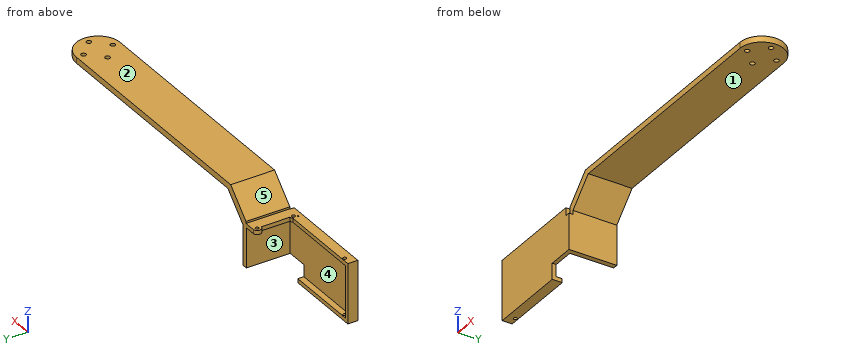
Autodesk Inventor part; units mm, degrees
ref_plane "YZ Plane" through (0, 0, 0) normal (1, 0, 0) x (0, 1, 0)
ref_plane "XZ Plane" through (0, 0, 0) normal (0, 1, 0) x (-1, 0, 0)
ref_plane "XY Plane" through (0, 0, 0) normal (0, 0, 1) x (1, 0, 0)
ref_plane "Plano de trabajo1" through (0, 0, 0) normal (0, 0, 1) x (1, 0, 0)
sketch "Boceto1" plane through (0, 0, 0) normal (0, 0, 1) x (1, 0, 0)
  circle A0 centre (10.9923, -7.35) radius 1.2028
  circle A1 centre (3.6423, 0) radius 1.2028
  circle A2 centre (18.3423, 0) radius 1.2028
  circle A3 centre (10.9923, 7.35) radius 1.2028
  circle A4 centre (10.9923, 0) radius 10.9823
  line L0 (10.9923, -10.9823) -> (-139.0077, -10.9823)
  line L1 (10.9923, 10.9823) -> (-139.0077, 10.9823)
  line L2 (-139.0077, 10.9823) -> (-139.0077, -10.9823)
  point P0 (0, 0)
  dimension "d0" = 150
  dimension "d1" = 150
extrude "Extrusión1" add sketch "Boceto1" along normal blind 3
sketch "Boceto2" plane through (0, 0, 3) normal (0, 0, 1) x (1, 0, 0)
  arc A0 (-129.1978, -5.6745) -> (-132.1454, -8.5217) centre (-128.1245, -9.7351) ccw
  circle A1 centre (-128.1245, 8.4649) radius 0.85 construction
  circle A2 centre (-128.1245, -9.7351) radius 0.7049 construction
  line L0 (-139.0305, -11.0697) -> (-267.2186, 10.8953)
  line L1 (-267.2186, -11.0694) -> (-117.2186, -11.0694)
  line L2 (-139.0305, 10.8953) -> (-139.0305, -11.0694)
  line L3 (-117.2186, 10.8953) -> (-267.2186, 10.8953)
  line L4 (-128.1245, -11.0697) -> (-128.1245, -0.0872)
  line L5 (-128.1245, -0.0872) -> (-128.1245, 9.0128)
  line L6 (-128.1245, -0.0872) -> (-128.1245, -9.1872)
  circle A3 centre (-128.1245, -9.1872) radius 0.85
  circle A4 centre (-128.1245, 9.0128) radius 0.85
  circle A5 centre (-128.1245, -9.1872) radius 1.8825
  circle A6 centre (-128.1245, 9.0128) radius 1.8821
  circle A7 centre (-128.1245, 9.0128) radius 0.85
  circle A8 centre (-128.1245, -9.1872) radius 0.85
  line L7 (-128.1245, 10.8953) -> (-139.0305, 10.8953)
  line L8 (-139.0077, 10.9823) -> (-139.0077, -10.9823)
  line L9 (-139.0077, -10.9823) -> (-139.0077, 10.9823)
  line L10 (-139.0077, 10.9823) -> (-139.0077, -10.9823)
  point P0 (0, 0)
  dimension "d4" = 10.9825
  dimension "d5" = 9.1
  dimension "d6" = 9.1
  dimension "d7" = 1.7
  dimension "d8" = 1.7
extrude "Extrusión2" cut sketch "Boceto2" against normal blind 3 contours A3 L4 | L4 A3 | A4
sketch "Boceto3" plane through (0, 0, 3) normal (0, 0, 1) x (1, 0, 0)
  circle A0 centre (-128.1245, -9.1872) radius 0.85
  circle A1 centre (-128.1245, 9.0128) radius 0.85
  line L0 (10.9923, 10.9823) -> (-139.0077, 10.9823)
  line L1 (-139.0077, 10.9823) -> (-139.0077, -10.9823)
  line L2 (-139.0077, -10.9823) -> (10.9923, -10.9823)
  arc A2 (10.9923, -10.9823) -> (10.9923, 10.9823) centre (10.9923, 0) ccw
  circle A3 centre (10.9923, -7.35) radius 1.2028
  circle A4 centre (3.6423, 0) radius 1.2028
  circle A5 centre (18.3423, 0) radius 1.2028
  circle A6 centre (10.9923, 7.35) radius 1.2028
  line L3 (-130.1442, 5.5225) -> (-129.5361, 14.2169)
  circle A7 centre (-128.1245, -9.1872) radius 1.7951
  circle A8 centre (-128.1245, 9.0128) radius 1.9695
  line L4 (-128.1245, -7.3921) -> (-128.1245, 7.0432)
  line L5 (-128.1245, -10.9823) -> (-128.1245, -18.0451)
  line L6 (-128.1245, -18.0451) -> (-142.6221, -18.554)
  line L7 (-142.6221, -18.554) -> (-141.7315, 12.8288)
  line L8 (-141.7315, 12.8288) -> (-128.1245, 12.4426)
  line L9 (-128.1245, 12.4426) -> (-128.1245, 10.9823)
  point P0 (0, 0)
extrude "Extrusión3" cut sketch "Boceto3" against normal blind 3 contours A8 L3 L0 | L3 A8 L4 A7 L2 L1 L0
sketch "Boceto4" plane through (0, 0, 0) normal (0, 0, -1) x (-1, 0, 0)
  arc A0 (128.1245, 7.0432) -> (128.1245, 10.9823) centre (128.1245, 9.0128) ccw
  line L0 (-10.9923, 10.9823) -> (128.1245, 10.9823)
  arc A1 (-10.9923, 10.9823) -> (-10.9923, -10.9823) centre (-10.9923, 0) ccw
  line L1 (128.1245, -10.9823) -> (-10.9923, -10.9823)
  arc A2 (128.1245, -10.9823) -> (128.1245, -7.3921) centre (128.1245, -9.1872) ccw
  line L2 (128.1245, -7.3921) -> (128.1245, 7.0432)
  circle A3 centre (128.1245, -9.1872) radius 0.85
  circle A4 centre (128.1245, 9.0128) radius 0.85
  circle A5 centre (-10.9923, -7.35) radius 1.2028
  circle A6 centre (-3.6423, 0) radius 1.2028
  circle A7 centre (-18.3423, 0) radius 1.2028
  circle A8 centre (-10.9923, 7.35) radius 1.2028
  line L3 (108.1857, 10.9823) -> (108.1857, -10.9823)
  point P0 (0, 0)
extrude "Extrusión4" add sketch "Boceto4" along normal blind 12 contours L2 A2 L1 L3 L0 A0
sketch "Boceto5" plane through (0, 0, 3) normal (0, 0, 1) x (1, 0, 0)
  line L0 (-108.1857, -10.9823) -> (-108.1857, 10.9823)
  circle A0 centre (10.9923, 7.35) radius 1.2028
  circle A1 centre (18.3423, 0) radius 1.2028
  circle A2 centre (3.6423, 0) radius 1.2028
  circle A3 centre (10.9923, -7.35) radius 1.2028
  arc A4 (-128.1245, 10.9823) -> (-128.1245, 7.0432) centre (-128.1245, 9.0128) ccw
  line L1 (-128.1245, 7.0432) -> (-128.1245, -7.3921)
  arc A5 (-128.1245, -7.3921) -> (-128.1245, -10.9823) centre (-128.1245, -9.1872) ccw
  line L2 (-128.1245, -10.9823) -> (10.9923, -10.9823)
  arc A6 (10.9923, -10.9823) -> (10.9923, 10.9823) centre (10.9923, 0) ccw
  line L3 (10.9923, 10.9823) -> (-128.1245, 10.9823)
  circle A7 centre (-128.1245, 9.0128) radius 0.85
  circle A8 centre (-128.1245, -9.1872) radius 0.85
  line L4 (-108.1857, 10.9823) -> (-111.1857, 10.9823)
  line L5 (-111.1857, 10.9823) -> (-111.1857, -10.9823)
  line L6 (-111.1857, -10.9823) -> (-108.1857, -10.9823)
  line L7 (-108.1857, -10.9823) -> (-108.1857, 10.9823)
  line L8 (10.9923, 10.9823) -> (-128.1245, 10.9823)
  line L9 (-122.3999, 10.9823) -> (-122.3999, -10.9823)
  point P0 (0, 0)
  dimension "d15" = 3
extrude "Extrusión5" cut sketch "Boceto5" against normal blind 13 contours L2 A5 L1 A4 L3 L9
chamfer "Chaflán1" distance 12 angle 45 1 edges at (-122.3999, 0, 3)
chamfer "Chaflán2" distance 12 angle 45 1 edges at (-108.1857, 0, -12)
sketch "Boceto6" plane through (0, 0, -12) normal (0, 0, -1) x (-1, 0, 0)
  line L0 (126.0445, -11.1372) -> (126.0445, 10.9228)
  line L1 (120.1857, -10.9823) -> (120.1857, 10.9823)
  line L2 (120.1857, -10.9823) -> (128.1245, -10.9823)
  line L3 (120.1857, 10.9823) -> (122.6857, 10.9823)
  line L4 (122.6857, 10.9823) -> (122.6857, -10.9823)
  line L5 (122.6857, -10.9823) -> (120.1857, -10.9823)
  line L6 (120.1857, -10.9823) -> (120.1857, 10.9823)
  point P0 (0, 0)
  dimension "d24" = 2.5
extrude "Extrusión6" add sketch "Boceto6" along normal blind 20
sketch "Boceto7" plane through (-128.1245, -10.9823, -10) normal (0, -1, 0) x (1, 0, 0)
  line L0 (19.9388, 10) -> (7.9388, -2)
  line L1 (19.9388, 10) -> (139.1168, 10)
  line L2 (139.1168, 10) -> (139.1168, 13)
  line L3 (17.7246, 13) -> (139.1168, 13)
  line L4 (5.7246, 1) -> (17.7246, 13)
  line L5 (5.7246, 1) -> (5.7246, 0)
  line L6 (5.7246, 0) -> (0, 0)
  line L7 (0, 0) -> (0, -2)
  line L8 (5.4388, -2) -> (0, -2)
  line L9 (5.4388, -2) -> (5.4388, -22)
  line L10 (7.9388, -22) -> (5.4388, -22)
  line L11 (7.9388, -2) -> (7.9388, -22)
  line L12 (7.9388, -2) -> (7.9388, -22)
  line L13 (5.4388, -22) -> (7.9388, -22)
  line L14 (7.9388, -22) -> (7.9388, -4)
  line L15 (7.9388, -4) -> (5.4388, -4)
  line L16 (5.4388, -4) -> (5.4388, -22)
  point P0 (128.1245, 10)
  point P1 (5.4388, -4)
  dimension "d27" = 18
extrude "Extrusión7" add sketch "Boceto7" along normal blind 2 contours L11 L10 L9 L15
sketch "Boceto8" plane through (-122.6857, -10.9823, -12) normal (-1, 0, 0) x (0, 0, 1)
  line L0 (0, 21.9646) -> (0, 0)
  line L1 (0, 21.9646) -> (-20, 21.9646)
  line L2 (-20, 21.9646) -> (-20, -2)
  line L3 (-2, -2) -> (-20, -2)
  line L4 (-2, 0) -> (-2, -2)
  line L5 (0, 0) -> (-2, 0)
  line L6 (-20, 0) -> (-2, 0)
  point P0 (12, 10.9823)
extrude "Extrusión8" add sketch "Boceto8" along normal blind 50 contours L4 L3 L2 L6
sketch "Boceto9" plane through (-120.1857, -12.9823, -14) normal (0, 0, 1) x (1, 0, 0)
  line L0 (-2.5, 2) -> (0, 2)
  line L1 (-2.5, 2) -> (-52.5, 2)
  line L2 (-52.5, 0) -> (-52.5, 2)
  line L3 (0, 0) -> (-52.5, 0)
  line L4 (0, 2) -> (0, 0)
  line L5 (-2.5, 0) -> (-52.5, 0)
  line L6 (-52.5, 0) -> (-52.5, 2)
  line L7 (-52.5, 2) -> (-2.5, 2)
  line L8 (-2.5, 2) -> (-2.5, 0)
  point P0 (120.1857, 12.9823)
extrude "Extrusión9" add sketch "Boceto9" along normal blind 4 contours L8 L3 L2 L1
sketch "Boceto10" plane through (0, 0, -32) normal (0, 0, -1) x (-1, 0, 0)
  line L0 (120.1857, 10.9823) -> (120.1857, -12.9823)
  line L1 (120.1857, -12.9823) -> (172.6857, -12.9823)
  line L2 (172.6857, -10.9823) -> (172.6857, -12.9823)
  line L3 (122.6857, -10.9823) -> (172.6857, -10.9823)
  line L4 (122.6857, 10.9823) -> (122.6857, -10.9823)
  line L5 (122.6857, 10.9823) -> (120.1857, 10.9823)
  line L6 (133.3495, -12.9823) -> (133.3495, -10.9823)
  line L7 (128.1245, -10.9823) -> (172.6857, -10.9823)
  point P0 (0, 0)
extrude "Extrusión10" add sketch "Boceto10" along normal blind 8 contours L6 L3 L2 L1
sketch "Boceto11" plane through (-172.6857, -10.9823, -10) normal (0, 1, 0) x (1, 0, 0)
  line L0 (50, 22) -> (50, 4)
  line L1 (50, 22) -> (39.3362, 22)
  line L2 (39.3362, 22) -> (39.3362, 30)
  line L3 (0, 30) -> (39.3362, 30)
  line L4 (0, 30) -> (0, 0)
  line L5 (44.5612, 0) -> (0, 0)
  line L6 (44.5612, 0) -> (44.5612, 2)
  line L7 (50, 2) -> (44.5612, 2)
  line L8 (50, 2) -> (50, 4)
  line L9 (39.3362, 22) -> (39.3362, 30)
  line L10 (39.3362, 30) -> (39.3362, 28)
  line L11 (39.3362, 28) -> (0, 28)
  line L12 (0, 28) -> (2, 28)
  line L13 (2, 28) -> (2, 0)
  line L14 (0, 0) -> (0, 30)
  line L15 (0, 0) -> (0, 2)
  line L16 (0, 2) -> (43.0714, 2)
  line L17 (43.0714, 2) -> (43.0714, 0)
  line L18 (44.5612, 0) -> (0, 0)
  point P0 (172.6857, -10)
  point P1 (2, 2)
  point P2 (39.3362, 28)
  dimension "d36" = 2
  dimension "d37" = 2
  dimension "d38" = 2
extrude "Extrusión11" add sketch "Boceto11" along normal blind 3 contours L11 L4 L3 L2 | L13 L16 L4 L11 | L16 L17 L5 L13 | L13 L5 L4 L16
sketch "Boceto12" plane through (0, 0, -40) normal (0, 0, -1) x (-1, 0, 0)
  circle A0 centre (168.3345, -9.2072) radius 0.85
  point P0 (0, 0)
extrude "Extrusión12" cut sketch "Boceto12" against normal blind 35
properties part number "femurAux"
The model under review builds one solid part; all positions refer to its coordinate system, in mm. Face numbers are marked on the shaded views. A direction names the side the tool comes from. Round coordinates to 2 decimals unless told otherwise and drop trailing zeros. Order: outer loops, then holes, each group sorted by start corner. A loop starts at its lowest first (then second) coordinate and runs counter-clockwise, first axis right, second up.
Item 1: Add section D-D, the plane x = -80. State the section outline as (y, z) points.
Working result:
outline: (-10.98, 0) - (10.98, 0) - (10.98, 3) - (-10.98, 3) - close
Item 2: Add section B-B, the plane x = -139. State the section outline as (y, z) points.
Working result:
outline: (-12.98, -40) - (-7.98, -40) - (-7.98, -38) - (-10.98, -38) - (-10.98, -12) - (-7.98, -12) - (-7.98, -10) - (-12.98, -10) - close
Item 3: Draft analysis for pull direction Z (two halves, no side actions). For the marked faces 3, 4 and 5, state which applies: released by +Z, released by -Z, zero draft, split by the parting line, or undercut.
Working result:
face 3: zero draft
face 4: undercut
face 5: released by +Z
Item 4: For pin 1 (8.5 mm diameter, centred on x = -153, z = -20.5, fed in from +Y); pin 2 (2.5 mm diameter, centred on x = -128.12, y = -9.19, fed in from +Z); pin 3 (8 mm diameter, centred on y = 6, z = -34, fed in from -X), all flat-tipped, find the tip position at first contact; note any pin that passes through.
Working result:
pin 1: stops at y = -10.98
pin 2: stops at z = -10
pin 3: stops at x = -122.69
Item 5: Machinability: for the marked faces 1 and 2, which of the approach directions +Z, -Z, +X, -X, +Y, -Y give a long, thin tool a straight path to every point of the face, cutting with its end or side? Answer none if there is none.
Working result:
face 1: -Z, +X, +Y, -Y
face 2: +Z, +X, -X, +Y, -Y
Item 6: To check wall thickness, follow probe 1 along Z at (x, y) = (-124, 7.5); probe 2 along X at (y, z) = (-10.25, -29); probe 3 along Z at (x, y) = (-74, 7.75). State the ranges of each line that lie inside material, in increasing order.
Working result:
probe 1: z = -12 to -10
probe 2: x = -172.69 to -170.69, -122.69 to -120.19
probe 3: z = 0 to 3
Item 7: Add section A-A, the plane z = -19. State the section outline as (x, y) points.
Working result:
outline: (-172.69, -12.98) - (-120.19, -12.98) - (-120.19, 10.98) - (-122.69, 10.98) - (-122.69, -10.98) - (-170.69, -10.98) - (-170.69, -7.98) - (-172.69, -7.98) - close
